The listing builds one solid part. Answer for the finished solid, in the listing's coordinates (mm). Give positions to 0.01 mm unless a question says otherwise; leave off trailing zeros. Loops run counter-clockwise (first coordinate to the right, second up) from the corner with the lowest first, then second, coordinate; pieces in that order, holes last. Notation, with made-up numbers: M -10,79 L 1,79 A22 ccw 1,96 Z; hole C 27,84.5 d5. An arc over 180 degrees is marked long. Use one line per item in the form item = value. Start each with the question number.
1. Straight lines are drawn through the part: line 1 (Z direction, x = -15, y = -1.95); line 2 (X direction, y = -1.2, z = -6.75); line 3 (X direction, y = -2.1, z = -5.25). For each, find the intervals that lie inside material, in ascending order. Write a range as from..to.
2. The part is cut by section A-A (x = -15). Write down the section's boundary in (y, z).
3. The mould has two halves that part along X. Classify faces 1 (the face through (-0.285, -0.301, -6.451)), 2 (the face through (-16.6, -1.5, -6.2)), 3 (the face through (-30, -1, -5)), 4 (the face through (-16, 0, -7)): released by +X, released by -X, zero draft, split by the parting line, or undercut.
4. The part is cut by section C-C (y = -1.65). Write down the section's boundary in (x, z).
5. The part is cut by section D-D (y = -0.5). Write down the section's boundary in (x, z).
6. The part is cut by section B-B (z = -5). Write down the section's boundary in (x, y).
from build123d import *

# Parameters (mm, degrees)
F0_R     = 2
F1_DEPTH = 3
F2_R     = 1


with BuildPart() as f1:
    # F0 (on Front) → F1 (new body)
    with BuildSketch(Plane.XZ):
        with BuildLine():
            ThreePointArc((0, -3), (-0.87868, -0.87868), (-3, 0))
            Line((-3, 0), (-30, 0))
            Line((-30, 0), (-30, -10))
            Line((-30, -10), (0, -10))
            Line((0, -10), (0, -3))
        make_face()
        with Locations((-15, -5)):
            Circle(F0_R, mode=Mode.SUBTRACT)
    extrude(amount=F1_DEPTH)

    # F2
    f2_edges = [f1.edges().sort_by_distance(p)[0] for p in [
        (-16.5, -3, 0),
        (-16.5, 0, 0),
    ]]
    fillet(f2_edges, radius=F2_R)


solid = f1.part
Derived:
q1.line_1 = -10..-7, -3..0
q1.line_2 = -30..-15.97, -14.03..0
q1.line_3 = -30..-16.98, -13.02..-0.01
q2.outline = M -3,-10 L 0,-10 L 0,-7 L -3,-7 Z; M -3,-3 L 0,-3 L 0,-1 A1 ccw -1,0 L -2,0 A1 ccw -3,-1 Z
q3.face_1 = released by +X
q3.face_2 = undercut
q3.face_3 = released by -X
q3.face_4 = zero draft
q4.outline = M -30,-10 L 0,-10 L 0,-3 A3 ccw -3,0 L -30,0 Z; hole C -15,-5 d4
q5.outline = M -30,-10 L -0.13,-10 L -0.13,-3 A2.87 ccw -3,-0.13 L -30,-0.13 Z; hole C -15,-5 d4
q6.outline = M -30,-3 L -17,-3 L -17,0 L -30,0 Z; M -13,-3 L -1,-3 A1 ccw 0,-2 L 0,-1 A1 ccw -1,0 L -13,0 Z
